from build123d import *

# Parameters (mm, degrees)
SKETCH_1_R      = 2.1
EXTRUDE_1_DEPTH = 3
FILLET_1_R      = 3


with BuildPart() as part:
    # 草图1 → 凸台-拉伸1 (new body)
    # profile 1 of 3: a face of its own
    with BuildSketch(Plane(origin=(0, 0, 0), x_dir=(1, 0, 0), z_dir=(0, 1, 0))):
        Polygon((35, -10), (35, 10), (-35, 10), (-35, -10), (-22.5, -10), (-10, -10), (-10, -22.5), (-10, -35), (10, -35), (10, -22.5), (10, -10), (22.5, -10), align=None)
        with Locations(Location((0, -25, 0), (0, 0, 270))):
            Circle(SKETCH_1_R, mode=Mode.SUBTRACT)
        with Locations(Location((-25, 0, 0), (0, 0, 270))):
            Circle(SKETCH_1_R, mode=Mode.SUBTRACT)
        with Locations(Location((0, 0, 0), (0, 0, 270))):
            Circle(SKETCH_1_R, mode=Mode.SUBTRACT)
        with Locations(Location((25, 0, 0), (0, 0, 270))):
            Circle(SKETCH_1_R, mode=Mode.SUBTRACT)
    # profile 2 of 3: a face of its own
    with BuildSketch(Plane(origin=(0, 0, 0), x_dir=(1, 0, 0), z_dir=(0, 1, 0))):
        Polygon((-10, -10), (-22.5, -10), (-10, -22.5), align=None)
    # profile 3 of 3: a face of its own
    with BuildSketch(Plane(origin=(0, 0, 0), x_dir=(1, 0, 0), z_dir=(0, 1, 0))):
        Polygon((10, -22.5), (22.5, -10), (10, -10), align=None)
    extrude(amount=EXTRUDE_1_DEPTH)

    # 圆角1
    fillet_1_edges = [part.edges().sort_by_distance(p)[0] for p in [
        (10, 1.5, 22.5),
        (10, 1.5, 35),
        (-10, 1.5, 35),
        (-10, 1.5, 22.5),
        (-22.5, 1.5, 10),
        (-35, 1.5, 10),
        (-35, 1.5, -10),
        (35, 1.5, -10),
        (35, 1.5, 10),
        (22.5, 1.5, 10),
    ]]
    fillet(fillet_1_edges, radius=FILLET_1_R)


solid = part.part
Geometry: final body of the model. Coordinates: model frame, mm. A direction names the side the tool comes from. Give positions to 0.01 mm unless a question says otherwise; leave off trailing zeros. Order: outer loops, then holes, each group sorted by start corner. A loop starts at its lowest first (then second) coordinate and runs counter-clockwise, first axis right, second up. Notation, with made-up numbers: (14, 7) -> (71, 7) arc R33 cw to (71, 36) -> close; hole circle Ø4 at (70, 67.25). An arc over 180 degrees is marked (long way). Answer as a JSON object with one key per item and string values.
Q1. Section D-D (x = -25). Output: boundary loops of the cut face in (y, z).
Entries:
{"outline": "(0, -10) -> (3, -10) -> (3, -2.1) -> (0, -2.1) -> close; (0, 2.1) -> (3, 2.1) -> (3, 10) -> (0, 10) -> close"}
Q2. Access query for faces 1 (the flat face through (-28, 1, 10)), 2 (the flat face through (0, 1, -10)). Directions: +Z, -Z, +X, -X, +Y, -Y. A direction counts if a zero-diameter tool reaches every point of the face in a straight line with its end or side. Return the directions, or none.
Entries:
{"face 1": "+Z, -X, +Y, -Y", "face 2": "-Z, +X, -X, +Y, -Y"}
Q3. Draft query along Z for faces 3 (the cylindrical face through (0.631, 1.479, 2.003)), 4 (the flat face through (10, 1, 28)), 5 (the cylindrical face through (-9.1, 1.52, 34.14)), 6 (the cylindrical face through (-0.8, 1.48, 26.94)). Return one class per face: released by +Z, released by -Z, zero draft, split by the parting line, or undercut.
Entries:
{"face 3": "undercut", "face 4": "zero draft", "face 5": "released by +Z", "face 6": "undercut"}
Q4. Material intervals for probe 1 along X at (y, z) = (2, 0); probe 2 along Z at (x, y) = (-1, 2.75); probe 3 along Z at (x, y) = (29, 0.3), sorted ascending.
Entries:
{"probe 1": "x = -35 to -27.1, -22.9 to -2.1, 2.1 to 22.9, 27.1 to 35", "probe 2": "z = -10 to -1.85, 1.85 to 23.15, 26.85 to 35", "probe 3": "z = -10 to 10"}
Q5. Section C-C (z = 0). Output: boundary loops of the cut face in (x, y), plus the area to 3 significant figures.
Entries:
{"outline": "(-35, 0) -> (-27.1, 0) -> (-27.1, 3) -> (-35, 3) -> close; (-22.9, 0) -> (-2.1, 0) -> (-2.1, 3) -> (-22.9, 3) -> close; (2.1, 0) -> (22.9, 0) -> (22.9, 3) -> (2.1, 3) -> close; (27.1, 0) -> (35, 0) -> (35, 3) -> (27.1, 3) -> close", "area": "172 mm^2"}
Q6. Section B-B (y = 0.9). Output: boundary loops of the cut face in (x, z).
Entries:
{"outline": "(-35, -7) arc R3 ccw to (-32, -10) -> (32, -10) arc R3 ccw to (35, -7) -> (35, 7) arc R3 ccw to (32, 10) -> (23.74, 10) arc R3 cw to (21.62, 10.88) -> (10.88, 21.62) arc R3 cw to (10, 23.74) -> (10, 32) arc R3 ccw to (7, 35) -> (-7, 35) arc R3 ccw to (-10, 32) -> (-10, 23.74) arc R3 cw to (-10.88, 21.62) -> (-21.62, 10.88) arc R3 cw to (-23.74, 10) -> (-32, 10) arc R3 ccw to (-35, 7) -> close; hole circle Ø4.2 at (-25, 0); hole circle Ø4.2 at (0, 0); hole circle Ø4.2 at (0, 25); hole circle Ø4.2 at (25, 0)"}
Q7. First-contact query: pin 1 (3.5 mm diameter, centred on x = 0, z = 0, fed in from +Y); pin 2 (1 mm diameter, centred on y = 2, z = 29, fed in from +X). Flat tips, straight axial feed; report the tip coordinate or a pass-through.
Entries:
{"pin 1": "passes through", "pin 2": "stops at x = 10"}
Q8. Section A-A (x = 0). Output: boundary loops of the cut face in (y, z).
Entries:
{"outline": "(0, -10) -> (3, -10) -> (3, -2.1) -> (0, -2.1) -> close; (0, 2.1) -> (3, 2.1) -> (3, 22.9) -> (0, 22.9) -> close; (0, 27.1) -> (3, 27.1) -> (3, 35) -> (0, 35) -> close"}
